from build123d import *

# Parameters (mm, degrees)
BOSS_EXTRUDE1_DEPTH = 3
SKETCH3_W           = 3
SKETCH3_H           = 15
BOSS_EXTRUDE2_DEPTH = 36
SKETCH5_W           = 15
SKETCH5_H           = 3
BOSS_EXTRUDE3_DEPTH = 10
SKETCH6_W           = 15
SKETCH6_H           = 3
BOSS_EXTRUDE4_DEPTH = 10
CUT_EXTRUDE1_DEPTH  = 3
FILLET1_R           = 5
FILLET2_R           = 1


with BuildPart() as part:
    # Sketch2 → Boss-Extrude1 (new body)
    with BuildSketch(Plane(origin=(0, 0, 0), x_dir=(1, 0, 0), z_dir=(0, 1, 0))):
        Polygon((32.5, 0), (0, 0), (-32.5, 0), (-32.5, -7.5), (32.5, -7.5), align=None)
        Polygon((-32.5, 0), (0, 0), (32.5, 0), (32.5, 7.5), (-32.5, 7.5), align=None)
    extrude(amount=BOSS_EXTRUDE1_DEPTH)

    # Sketch3 → Boss-Extrude2 (add)
    with BuildSketch(Plane.XZ):
        Polygon((-29.5, 7.5), (-32.5, 7.5), (-32.5, -7.5), align=None)
        Polygon((-29.5, -7.5), (-29.5, 7.5), (-32.5, -7.5), align=None)
        with Locations((31, 0)):
            Rectangle(SKETCH3_W, SKETCH3_H)
    extrude(amount=BOSS_EXTRUDE2_DEPTH)

    # Sketch5 → Boss-Extrude3 (add)
    with BuildSketch(Plane(origin=(32.5, 0, 0), x_dir=(0, 0, -1), z_dir=(1, 0, 0))):
        with Locations((0, -34.5)):
            Rectangle(SKETCH5_W, SKETCH5_H)
    extrude(amount=BOSS_EXTRUDE3_DEPTH)

    # Sketch6 → Boss-Extrude4 (add)
    with BuildSketch(Plane.ZY.offset(32.5)):
        with Locations((0, -34.5)):
            Rectangle(SKETCH6_W, SKETCH6_H)
    extrude(amount=BOSS_EXTRUDE4_DEPTH)

    # Sketch7 → Cut-Extrude1 (cut)
    with BuildSketch(Plane(origin=(0, -33, 0), x_dir=(1, 0, 0), z_dir=(0, 1, 0))):
        with BuildLine():
            ThreePointArc((-35.5, 0), (-36.556284149, 1.763349198), (-38.609400392, 1.664100589))
            Line((-38.609400392, 1.664100589), (-36.390599608, -1.664100589))
            ThreePointArc((-36.390599608, -1.664100589), (-35.736650802, -0.943715851), (-35.5, 0))
        make_face()
        with BuildLine():
            Line((-36.390599608, -1.664100589), (-38.609400392, 1.664100589))
            ThreePointArc((-38.609400392, 1.664100589), (-39.164100589, -1.109400392), (-36.390599608, -1.664100589))
        make_face()
        with BuildLine():
            ThreePointArc((36.390599608, 1.664100589), (35.835899411, -1.109400392), (38.609400392, -1.664100589))
            Line((38.609400392, -1.664100589), (36.390599608, 1.664100589))
        make_face()
        with BuildLine():
            Line((36.390599608, 1.664100589), (38.609400392, -1.664100589))
            ThreePointArc((38.609400392, -1.664100589), (39.263349198, -0.943715851), (39.5, 0))
            ThreePointArc((39.5, 0), (38.443715851, 1.763349198), (36.390599608, 1.664100589))
        make_face()
    extrude(amount=-CUT_EXTRUDE1_DEPTH, mode=Mode.SUBTRACT)

    # Fillet1
    fillet1_edges = [part.edges().sort_by_distance(p)[0] for p in [
        (32.5, 3, 0),
        (-32.5, 3, 0),
    ]]
    fillet(fillet1_edges, radius=FILLET1_R)

    # Fillet2
    fillet2_edges = [part.edges().sort_by_distance(p)[0] for p in [
        (-38.609400392, -33, -1.664100589),
        (38.609400392, -33, 1.664100589),
    ]]
    fillet(fillet2_edges, radius=FILLET2_R)


solid = part.part
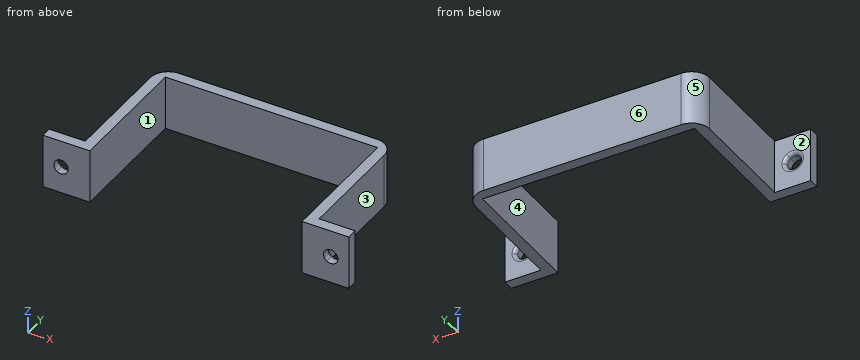
CAD build for the part. Positions are in the model's coordinates, mm. Face numbers are marked on the shaded views. A direction names the side the tool comes from. Round coordinates to 2 decimals unless told otherwise and drop trailing zeros. Order: outer loops, then holes, each group sorted by start corner. A loop starts at its lowest first (then second) coordinate and runs counter-clockwise, first axis right, second up. Notation, with made-up numbers: (7, 73.5) - (35, 73.5) arc R34 cw to (35, 107.5) - close; hole circle Ø3 at (-8, 4.5). An arc over 180 degrees is marked (long way). Return JSON: item names as keys, results as strings.
(1) Pin check, flat tips, straight feed: pin 1 Ø3 at (y, z) = (-26, 5.5) entering from +X; pin 2 Ø7.5 at (y, z) = (-11, -3) entering from -X; pin 3 Ø3 at (x, z) = (-30.5, 0) entering from +Y. Stop position of each tip, or through.
Answer key:
{"pin 1": "stops at x = 32.5", "pin 2": "stops at x = -32.5", "pin 3": "stops at y = 2.77"}
(2) Cut at D-D (x = -30.5). Give the cut face in (y, z), then the cut area to 3 significant figures.
Answer key:
{"outline": "(-36, -7.5) - (2, -7.5) - (2, 7.5) - (-36, 7.5) - close", "area": "570 mm^2"}
(3) Cut at B-B (z = -6.25). Give the cut face in (x, y).
Answer key:
{"outline": "(-42.5, -36) - (-29.5, -36) - (-29.5, 0) - (29.5, 0) - (29.5, -36) - (42.5, -36) - (42.5, -33) - (32.5, -33) - (32.5, -2) arc R5 ccw to (27.5, 3) - (-27.5, 3) arc R5 ccw to (-32.5, -2) - (-32.5, -33) - (-42.5, -33) - close"}
(4) Wall check: probe 1 along X at (y, z) = (-30, 2.25); probe 2 along Y at (x, z) = (24.5, 4.75); probe 3 along Y at (x, z) = (34, -0.5). Give the ranges that are in metal, low to high. Write a range as from..to.
Answer key:
{"probe 1": "x = -32.5..-29.5, 29.5..32.5", "probe 2": "y = 0..3", "probe 3": "y = -36..-33"}
(5) Tool access for the marked faces 1, 2 and 3: list every direction of +Z, -Z, +X, -X, +Y, -Y with a clear straight run to the whole face (end or side of a thin tool).
Answer key:
{"face 1": "+Z, -Z, -Y", "face 2": "+Z, -Z, -X, +Y", "face 3": "+Z, -Z, +X, +Y"}
(6) Pull direction X, two halves, no side cores. Call the marked faces 4, 5 and 6: +X half, -X half, draft (parallel to the pull), parting line (faces both ways), or undercut.
Answer key:
{"face 4": "undercut", "face 5": "-X half", "face 6": "draft"}
(7) Cut at C-C (x = -15.5). Give the cut face in (y, z), then the cut area to 3 significant figures.
Answer key:
{"outline": "(0, -7.5) - (3, -7.5) - (3, 7.5) - (0, 7.5) - close", "area": "45.0 mm^2"}
(8) Cut at A-A (y = -22). Give the cut face in (x, z), then the cut area to 3 significant figures.
Answer key:
{"outline": "(-32.5, -7.5) - (-29.5, -7.5) - (-29.5, 7.5) - (-32.5, 7.5) - close; (29.5, -7.5) - (32.5, -7.5) - (32.5, 7.5) - (29.5, 7.5) - close", "area": "90.0 mm^2"}
